Build history of the part. All positions in model axes, mm. A direction names the side the tool comes from. Give positions to 0.01 mm unless a question says otherwise; leave off trailing zeros. Write each loop counter-clockwise with the first axis right and the second up, starting at its lowest first coordinate (ties: lowest second). Pieces come first, ordered by that corner, then holes. Notation, with made-up numbers: M -37,-25.5 L 0,-25.5 A24 ccw 0,3.5 Z; hole C 81,57.5 d1. An arc over 180 degrees is marked long. Return JSON: item names as keys, results as strings. Group by question number.
Q1. Flat gauge pins, fed straight in: pin 1 Ø1.5 at (x, z) = (10.5, 7) entering from +Y; pin 2 Ø1.5 at (x, z) = (5.5, 2.5) entering from +Y; pin 3 Ø0.9 at (x, z) = (1.5, 3.5) entering from +Y; pin 4 Ø1.5 at (x, z) = (5.5, 3) entering from -Y. Where does each tip first touch, or does it go through?
Q2. Tool access for faces 1 (the flat face through (24.959, -25, 3)), 2 (the flat face through (3, -56.324, 3)), 3 (the flat face through (-18.3, -24.7, 5)): list every direction of +Z, -Z, +X, -X, +Y, -Y with a clear straight run to the whole face (end or side of a thin tool).
Q3. Band-saw the part on D-D, the plane x = -20. Give the cut face in (y, z), then the cut area to 3 significant figures.
Q4. Wall check: probe 1 along X at (y, z) = (-12, 2.5); probe 2 along X at (y, z) = (-8, 0.5); probe 3 along X at (y, z) = (24, 6.25). Give the ranges that are in metal, low to high.
Q5. Band-saw the part on A-A, the plane y = -33.5. Give the cut face in (x, z).
Q6. Band-saw the part on B-B, the plane z = 4. Give the cut face in (x, y), then the cut area to 3 significant figures.
Q7. Pull direction Y, two halves, no side cores. Call faces 4 (the flat face through (3, 5.676, 3)), 5 (the flat face through (-19.041, -25, 3)), 6 (the flat face through (3, 6.676, 3)): +Y half, -Y half, draft (parallel to the pull), parting line (faces both ways), or undercut.
Q8. Band-saw the part on C-C, the plane x = 2.5. Give the cut face in (y, z), then the cut area to 3 significant figures.
from build123d import *

# Parameters (mm, degrees)
SKETCH_W        = 70
SKETCH_H        = 90
PAD_DEPTH       = 2
SKETCH001_W     = 43
SKETCH001_H     = 61
POCKET_DEPTH    = 2
SKETCH002_W     = 45
SKETCH002_H     = 63
PAD001_DEPTH    = 3
SKETCH003_W     = 43
SKETCH003_H     = 61
POCKET001_DEPTH = 3
SKETCH004_W     = 2
SKETCH004_H     = 90
PAD002_DEPTH    = 6
SKETCH005_W     = 90
SKETCH005_H     = 1
PAD003_DEPTH    = 0.5
SKETCH006_W     = 90
SKETCH006_H     = 1
PAD004_DEPTH    = 0.5


with BuildPart() as part:
    # Sketch → Pad (new body)
    with BuildSketch(Plane.XY):
        with Locations((3.459163, -17.324317)):
            Rectangle(SKETCH_W, SKETCH_H)
    extrude(amount=PAD_DEPTH)

    # Sketch001 (on Face6 of Pad) → Pocket (cut)
    with BuildSketch(Plane.XY.offset(2)):
        with Locations((3.459163, -24.824317)):
            Rectangle(SKETCH001_W, SKETCH001_H)
    extrude(amount=-POCKET_DEPTH, mode=Mode.SUBTRACT)

    # Sketch002 (on Face5 of Pocket) → Pad001 (join)
    with BuildSketch(Plane.XY.offset(2)):
        with Locations((3.459163, -24.824317)):
            Rectangle(SKETCH002_W, SKETCH002_H)
    extrude(amount=PAD001_DEPTH)

    # Sketch003 (on Face16 of Pad001) → Pocket001 (cut)
    with BuildSketch(Plane.XY.offset(5)):
        with Locations((3.459163, -24.824317)):
            Rectangle(SKETCH003_W, SKETCH003_H)
    extrude(amount=-POCKET001_DEPTH, mode=Mode.SUBTRACT)

    # Sketch004 (on Face5 of Pocket001) → Pad002 (join)
    with BuildSketch(Plane.XY.offset(2)):
        with Locations((-30.540837, -17.324317)):
            Rectangle(SKETCH004_W, SKETCH004_H)
        with Locations((37.459163, -17.324317)):
            Rectangle(SKETCH004_W, SKETCH004_H)
    extrude(amount=PAD002_DEPTH)

    # Sketch005 (on Face17 of Pad002) → Pad003 (join)
    with BuildSketch(Plane(origin=(36.459163, 0, 0), x_dir=(0, -1, 0), z_dir=(-1, 0, 0))):
        with Locations((17.324317, 7.5)):
            Rectangle(SKETCH005_W, SKETCH005_H)
    extrude(amount=PAD003_DEPTH)

    # Sketch006 (on Face15 of Pad003) → Pad004 (join)
    with BuildSketch(Plane.YZ.offset(-29.540837)):
        with Locations((-17.324317, 7.5)):
            Rectangle(SKETCH006_W, SKETCH006_H)
    extrude(amount=PAD004_DEPTH)


solid = part.part
From the geometry:
{
 "1": {"pin 1": "passes through", "pin 2": "stops at y = 27.68", "pin 3": "stops at y = 6.68", "pin 4": "stops at y = -56.32"},
 "2": {"face 1": "+Z, -Z", "face 2": "+Z, -Y", "face 3": "+Z, +Y, -Y"},
 "3": {"outline": "M -62.32,0 L 27.68,0 L 27.68,2 L -62.32,2 Z", "area": "180 mm^2"},
 "4": {"probe 1": "x = -31.54 to -29.54, -19.04 to -18.04, 24.96 to 25.96, 36.46 to 38.46", "probe 2": "x = -31.54 to -18.04, 24.96 to 38.46", "probe 3": "x = -31.54 to -29.54, 36.46 to 38.46"},
 "5": {"outline": "M -31.54,0 L -18.04,0 L -18.04,5 L -19.04,5 L -19.04,2 L -29.54,2 L -29.54,7 L -29.04,7 L -29.04,8 L -31.54,8 Z; M 24.96,0 L 38.46,0 L 38.46,8 L 35.96,8 L 35.96,7 L 36.46,7 L 36.46,2 L 25.96,2 L 25.96,5 L 24.96,5 Z"},
 "6": {"outline": "M -31.54,-62.32 L -29.54,-62.32 L -29.54,27.68 L -31.54,27.68 Z; M -19.04,-56.32 L 25.96,-56.32 L 25.96,6.68 L -19.04,6.68 Z; M 36.46,-62.32 L 38.46,-62.32 L 38.46,27.68 L 36.46,27.68 Z; hole M -18.04,-55.32 L 24.96,-55.32 L 24.96,5.68 L -18.04,5.68 Z", "area": "572 mm^2"},
 "7": {"face 4": "undercut", "face 5": "draft", "face 6": "+Y half"},
 "8": {"outline": "M -62.32,0 L -55.32,0 L -55.32,5 L -56.32,5 L -56.32,2 L -62.32,2 Z; M 5.68,0 L 27.68,0 L 27.68,2 L 6.68,2 L 6.68,5 L 5.68,5 Z", "area": "64.0 mm^2"}
}
